Can you work these out from the model? Positions are in its coordinate system, mm. A direction names the side the tool comes from. Round coordinates to 2 decimals unless told otherwise and drop trailing zeros. Loops run counter-clockwise (first coordinate to the right, second up) from the corner with the lowest first, then second, coordinate; pieces in that order, holes last.
```python
from build123d import *

# Parameters (mm, degrees)
F1_DEPTH = 120
F2_R     = 7
F3_DEPTH = 25


with BuildPart() as f1:
    # F0 (on Front) → F1 (new body)
    with BuildSketch(Plane.XZ):
        with BuildLine():
            ThreePointArc((-71.811404, 0), (-71.49001, 0.116978), (-71.319, 0.413176))
            Line((-71.319, 0.413176), (-58.519957, 73.000157))
            ThreePointArc((-58.519957, 73.000157), (-56.125816, 77.146931), (-51.626303, 78.78462))
            Line((-51.626303, 78.78462), (51.626303, 78.78462))
            ThreePointArc((51.626303, 78.78462), (56.125816, 77.146931), (58.519957, 73.000157))
            Line((58.519957, 73.000157), (71.319, 0.413176))
            ThreePointArc((71.319, 0.413176), (71.49001, 0.116978), (71.811404, 0))
            Line((71.811404, 0), (77.903964, 0))
            ThreePointArc((77.903964, 0), (78.286986, 0.178606), (78.396368, 0.586824))
            Line((78.396368, 0.586824), (64.393654, 80.000157))
            ThreePointArc((64.393654, 80.000157), (61.999513, 84.146931), (57.5, 85.78462))
            Line((57.5, 85.78462), (-57.5, 85.78462))
            ThreePointArc((-57.5, 85.78462), (-61.999513, 84.146931), (-64.393654, 80.000157))
            Line((-64.393654, 80.000157), (-78.396368, 0.586824))
            ThreePointArc((-78.396368, 0.586824), (-78.286986, 0.178606), (-77.903964, 0))
            Line((-77.903964, 0), (-71.811404, 0))
        make_face()
    extrude(amount=F1_DEPTH)

    # F2 (on face) → F3 (cut)
    with BuildSketch(Plane.XY.offset(85.78462)):
        with Locations((0, -60)):
            Circle(F2_R)
    extrude(amount=-F3_DEPTH, mode=Mode.SUBTRACT)


solid = f1.part
```
(1) Suppose I cut it at C-C (z = 35). Write out the boundary of the cut face in (x, y).
(2) For pin 1 (5 mm diameter, centred on x = 9, y = -93, fed in from -Z); pin 2 (8.5 mm diameter, centred on x = 0, y = -60, fed in from -Z); pin 3 (1 mm diameter, centred on y = -23, z = 58.5, fed in from -X), each with a flat end and sliding along its axis, tell me the tip position at first contact or that it passes through.
(3) We'd pull the mould along X, two halves only. Please class faces 3 (the flat face through (-65.01, -59.16, 36.2)), 4 (the flat face through (64.83, -59.16, 37.21)), 5 (the flat face through (-71.297, -59.16, 40.849)), 6 (the flat face through (-75, -59, 0)): released by +X, released by -X, zero draft, split by the parting line, or undercut.
(4) If I drill on line 1 (Y direction, x = 0, z = 83.75); line 2 (Z direction, x = -50.5, y = -58); line 3 (X direction, y = -58, z = 77), over which ranges is the centre line in solid material (lowest first)?
(5) Suppose I cut it at B-B (y = -60). Write out the boundary of the cut face in (x, z).
(6) Suppose I cut it at A-A (x = 0). Write out the boundary of the cut face in (y, z).
(7) Which directions (+Z, -Z, +X, -X, +Y, -Y) give clear straight access to the entire face, cutting with the end or side of a thin tool? Please do faces 1 (the cylindrical face through (-56.18, -59.16, 77.1)), 2 (the cylindrical face through (-0.91, -53.06, 82.33)).
(8) Suppose I cut it at D-D (x = 30). Write out the boundary of the cut face in (y, z), then the cut area to 3 significant figures.
Check result:
1. outline: (-72.33, -120) - (-65.22, -120) - (-65.22, 0) - (-72.33, 0) - close; (65.22, -120) - (72.33, -120) - (72.33, 0) - (65.22, 0) - close
2. pin 1: stops at z = 78.78
2. pin 2: passes through
2. pin 3: stops at x = -68.27
3. face 3: undercut
3. face 4: undercut
3. face 5: released by -X
3. face 6: zero draft
4. line 1: y = -120 to -67, -53 to 0
4. line 2: z = 78.78 to 85.78
4. line 3: x = -64.92 to -56.3, 56.3 to 64.92
5. outline: (-78.4, 0.59) arc R0.5 ccw to (-77.9, 0) - (-71.81, 0) arc R0.5 ccw to (-71.32, 0.41) - (-58.52, 73) arc R7 cw to (-51.63, 78.78) - (-7, 78.78) - (-7, 85.78) - (-57.5, 85.78) arc R7 ccw to (-64.39, 80) - close; (7, 78.78) - (51.63, 78.78) arc R7 cw to (58.52, 73) - (71.32, 0.41) arc R0.5 ccw to (71.81, 0) - (77.9, 0) arc R0.5 ccw to (78.4, 0.59) - (64.39, 80) arc R7 ccw to (57.5, 85.78) - (7, 85.78) - close
6. outline: (-120, 78.78) - (-67, 78.78) - (-67, 85.78) - (-120, 85.78) - close; (-53, 78.78) - (0, 78.78) - (0, 85.78) - (-53, 85.78) - close
7. face 1: -Z, +Y, -Y
7. face 2: +Z, -Z
8. outline: (-120, 78.78) - (0, 78.78) - (0, 85.78) - (-120, 85.78) - close
8. area: 840 mm2
